The drawing under review shows one solid part. Ordinate dimensions are in mm from its lowest x, y, z. A direction names the side the tool comes from. Give positions to 0.01 mm unless a question says otherwise; leave off trailing zeros. Order: outer loops, then holes, each group sorted by start corner. A loop starts at its lowest first (then second) coordinate and runs counter-clockwise, first axis right, second up. Notation, with made-up numbers: (9, 23.25) -> (28, 23.25) arc R8 ccw to (28, 27.25) -> close; hole circle Ø11 at (-32.5, -6.75). An arc over 180 degrees is marked (long way). One line per item, written item: value. Start each with the question number.
1) Consider section D-D (z = 5.5). State the section outline as (x, y) points.
2) Consider section B-B (z = 55). State the section outline as (x, y) points, plus the area to 3 significant figures.
3) For pin 1 (16 mm diameter, centred on x = 50.5, z = 13, fed in from -Y); pin 2 (4 mm diameter, centred on y = 15, z = 17.5, fed in from +X), all flat-tipped, find the tip position at first contact; note any pin that passes through.
4) Consider section C-C (y = 37.5). State the section outline as (x, z) points.
5) Wall thickness on line 1 along Z through (x, y) = (33.5, 10.5); line 2 along Y through (x, z) = (34, 15.5): over which ranges is each line inside the solid? List them lowest first. Write a range as from..to.
6) The part is to be moulded in two halves that separate along Y. For the marked faces 1, 2, 3 and 4, say which applies: released by +Y, released by -Y, zero draft, split by the parting line, or undercut.
7) Consider section A-A (x = 50). State the section outline as (y, z) points.
8) Tool access review of the marked faces 5, 6, 7, 8 and 9: name each direction out of +Z, -Z, +X, -X, +Y, -Y from which nothing blocks a thin tool from reaching the whole face with its end or side.
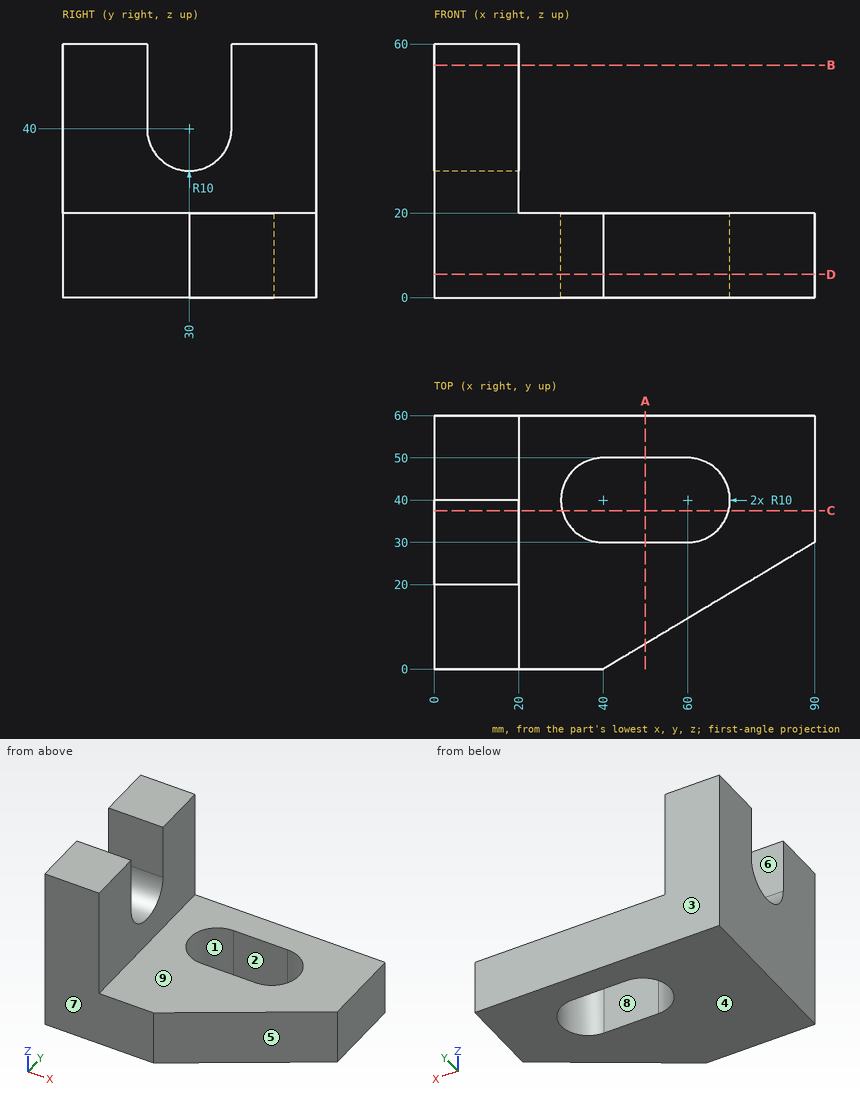
Checked values:
1. outline: (0, 0) -> (40, 0) -> (90, 30) -> (90, 60) -> (0, 60) -> close; hole (40, 30) -> (60, 30) arc R10 ccw to (60, 50) -> (40, 50) arc R10 ccw to start
2. outline: (0, 0) -> (20, 0) -> (20, 20) -> (0, 20) -> close; (0, 40) -> (20, 40) -> (20, 60) -> (0, 60) -> close
2. area: 800 mm^2
3. pin 1: stops at y = 1.5
3. pin 2: stops at x = 68.33
4. outline: (0, 0) -> (30.32, 0) -> (30.32, 20) -> (20, 20) -> (20, 33.39) -> (0, 33.39) -> close; (69.68, 0) -> (90, 0) -> (90, 20) -> (69.68, 20) -> close
5. line 1: z = 0..20
5. line 2: y = 0..32, 48..60
6. face 1: undercut
6. face 2: undercut
6. face 3: released by +Y
6. face 4: zero draft
7. outline: (6, 0) -> (30, 0) -> (30, 20) -> (6, 20) -> close; (50, 0) -> (60, 0) -> (60, 20) -> (50, 20) -> close
8. face 5: +Z, -Z, +X, -Y
8. face 6: +Z, +X, -X
8. face 7: +Z, -Z, +X, -X, -Y
8. face 8: +Z, -Z
8. face 9: +Z, +X, +Y, -Y
